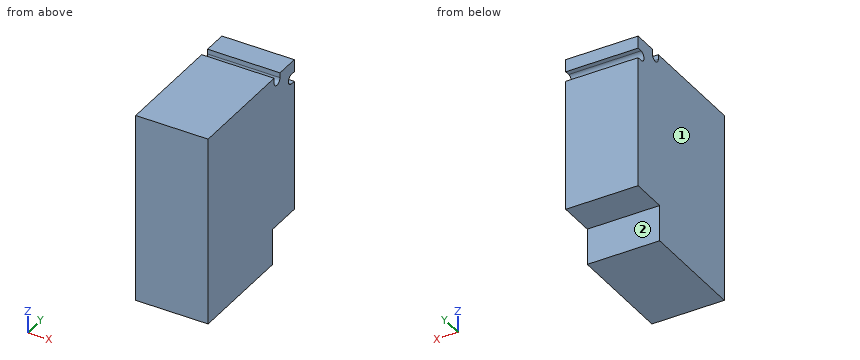
from build123d import *

# Parameters (mm, degrees)
F1_DEPTH = 12.7


with BuildPart() as f1:
    # F0 (on Right) → F1 (new body)
    with BuildSketch(Plane.YZ):
        with BuildLine():
            Line((-15.011845, 36.838097), (-34.468245, 36.838097))
            Line((-34.468245, 36.838097), (-34.468245, 3.500597))
            Line((-34.468245, 3.500597), (-15.418245, 3.500597))
            Line((-15.418245, 3.500597), (-15.418245, 9.850597))
            Line((-15.418245, 9.850597), (-9.068245, 9.850597))
            Line((-9.068245, 9.850597), (-9.068245, 32.926497))
            Line((-9.068245, 32.926497), (-9.931845, 32.926497))
            ThreePointArc((-9.931845, 32.926497), (-10.795445, 33.790097), (-9.931845, 34.653697))
            Line((-9.931845, 34.653697), (-9.068245, 34.653697))
            Line((-9.068245, 34.653697), (-9.068245, 36.838097))
            Line((-9.068245, 36.838097), (-13.284645, 36.838097))
            Line((-13.284645, 36.838097), (-13.284645, 35.974497))
            ThreePointArc((-13.284645, 35.974497), (-14.148245, 35.110897), (-15.011845, 35.974497))
            Line((-15.011845, 35.974497), (-15.011845, 36.838097))
        make_face()
    extrude(amount=F1_DEPTH)


solid = f1.part
Work out the finished part from the listing and answer in its coordinate system (mm). Face numbers are marked on the shaded views. A direction names the side the tool comes from. Give positions to 0.01 mm unless a question says otherwise; leave off trailing zeros. Loops run counter-clockwise (first coordinate to the right, second up) from the corner with the lowest first, then second, coordinate; pieces in that order, holes last. Notation, with made-up numbers: (56.5, -20.75) - (69.5, -20.75) arc R15 cw to (69.5, -3.75) - close; hole circle Ø10 at (8, 63). An arc over 180 degrees is marked (long way). Answer in a Markdown table with one row per item. Add a question column.
Q1. The part is cut by section B-B (y = -12). Determine the outline of the cut face in (x, z), and give its area (3 significant figures).
Q2. Each of these flat-tipped pins is pushed along its axis until it touches: P1, Ø1.9, axis at x = 6.5, z = 5, coming from the +Y side; P2, Ø7, axis at x = 9, y = -11, coming from the -Z side. Where does it stop, or does it pass through?
Q3. The part is cut by section A-A (x = 4.75). Determine the outline of the cut face in (y, z), and give its area (3 significant figures).
Q4. A tool of negligible diameter and unlimited length cuts with its end or side. For the marked faces 1 and 2, from which of +Z, -Z, +X, -X, +Y, -Y can it reach the whole face along a straight path? Write none if from no direction.
Q5. The part is cut by section C-C (z = 7.5). Determine the outline of the cut face in (x, y), and give its area (3 significant figures).
Q6. Consider line 1 along Z through (x, y) = (5.25, -10); line 2 along Y through (x, z) = (1, 5); line 3 along Z through (x, y) = (2, -12.75). Determine where each line is inside the solid, lowest interval first.
Solution:
| question | item | result |
|---|---|---|
| 1 | outline | (0, 9.85) - (12.7, 9.85) - (12.7, 36.84) - (0, 36.84) - close |
| 1 | area | 343 mm² |
| 2 | P1 | stops at y = -15.42 |
| 2 | P2 | stops at z = 9.85 |
| 3 | outline | (-34.47, 3.5) - (-15.42, 3.5) - (-15.42, 9.85) - (-9.07, 9.85) - (-9.07, 32.93) - (-9.93, 32.93) arc R0.86 cw to (-9.93, 34.65) - (-9.07, 34.65) - (-9.07, 36.84) - (-13.28, 36.84) - (-13.28, 35.97) arc R0.86 cw to (-15.01, 35.97) - (-15.01, 36.84) - (-34.47, 36.84) - close |
| 3 | area | 801 mm² |
| 4 | face 1 | +Z, -Z, -X, +Y, -Y |
| 4 | face 2 | -Z, +X, -X, +Y |
| 5 | outline | (0, -34.47) - (12.7, -34.47) - (12.7, -15.42) - (0, -15.42) - close |
| 5 | area | 242 mm² |
| 6 | line 1 | z = 9.85 to 32.93, 34.65 to 36.84 |
| 6 | line 2 | y = -34.47 to -15.42 |
| 6 | line 3 | z = 9.85 to 36.84 |
